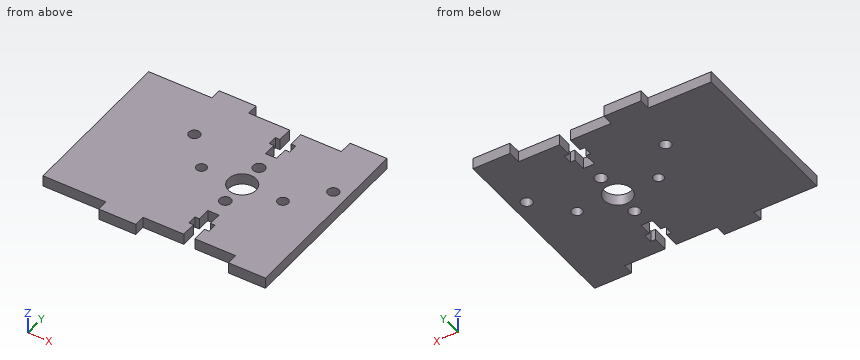
```python
from build123d import *

# Parameters (mm, degrees)
MODEL_R             = 3.750000001
MODEL_R_2           = 1.500000002
MODEL_R_3           = 1.353150001
MODEL_R_4           = 1.598250001
MODEL_R_5           = 1.533250001
MODEL_R_6           = 1.426350001
BOSS_EXTRUDE1_DEPTH = 3


with BuildPart() as part:
    # Model → Boss-Extrude1 (new body)
    with BuildSketch(Plane.XY):
        Polygon((58.24, 47.9), (61.24, 47.9), (61.24, 51.4001), (62.49, 51.4001), (62.49, 53.9001), (61.24, 53.9001), (61.24, 57.9), (72.24, 57.9), (72.24, 61.449728443), (82.24, 61.449728443), (82.24, 57.9), (82.24, 13.9), (82.24, 10.9), (72.24, 10.9), (72.24, 13.9), (61.24, 13.9), (61.24, 17.9), (62.49, 17.9), (62.49, 20.4), (61.24, 20.4), (61.24, 23.9), (58.24, 23.9), (58.24, 20.4), (56.99, 20.4), (56.99, 17.9), (58.24, 17.9), (58.24, 13.9), (47.24, 13.9), (47.24, 10.9), (37.24, 10.9), (37.24, 13.9), (20.24, 13.9), (20.24, 57.9), (37.24, 57.9), (37.24, 60.9), (47.24, 60.9), (47.24, 57.9), (58.24, 57.9), (58.24, 53.9001), (56.99, 53.9001), (56.99, 51.4001), (58.24, 51.4001), align=None)
        with Locations((59.739999999, 35.899999999)):
            Circle(MODEL_R, mode=Mode.SUBTRACT)
        with Locations((40.989999998, 44.899999998)):
            Circle(MODEL_R_2, mode=Mode.SUBTRACT)
        with Locations((48.73995, 35.90005)):
            Circle(MODEL_R_3, mode=Mode.SUBTRACT)
        with Locations((59.73995, 42.90005)):
            Circle(MODEL_R_4, mode=Mode.SUBTRACT)
        with Locations((59.73995, 28.90005)):
            Circle(MODEL_R_5, mode=Mode.SUBTRACT)
        with Locations((70.73995, 35.90005)):
            Circle(MODEL_R_6, mode=Mode.SUBTRACT)
        with Locations((78.489999998, 44.899999998)):
            Circle(MODEL_R_2, mode=Mode.SUBTRACT)
    extrude(amount=BOSS_EXTRUDE1_DEPTH)


solid = part.part
```
The model under review builds one solid part; all positions refer to its coordinate system, in mm. Round coordinates to 2 decimals unless told otherwise and drop trailing zeros. Loops run counter-clockwise (first coordinate to the right, second up) from the corner with the lowest first, then second, coordinate; pieces in that order, holes last. Notation, with made-up numbers: M 10,82 L 30,82 A19 ccw 30,90 Z; hole C 67.25,-5.75 d4. An arc over 180 degrees is marked long. Put each result on its own line as item: value.
Q1. To check wall thickness, follow L1, parallel to X at y = 35.9, z = 1.35; L2, parallel to X at y = 44.9, z = 0.85; L3, parallel to X at y = 22, z = 2.3. State the ranges of each line that lie inside material, in increasing order.
Result set:
L1: x = 20.24 to 47.39, 50.09 to 55.99, 63.49 to 69.31, 72.17 to 82.24
L2: x = 20.24 to 39.49, 42.49 to 76.99, 79.99 to 82.24
L3: x = 20.24 to 58.24, 61.24 to 82.24
Q2. Consider section B-B, the plane x = 59.74. Give the boundary of the cut face in (y, z), then the cut area to 3 significant figures.
Result set:
outline: M 23.9,0 L 27.37,0 L 27.37,3 L 23.9,3 Z; M 30.43,0 L 32.15,0 L 32.15,3 L 30.43,3 Z; M 39.65,0 L 41.3,0 L 41.3,3 L 39.65,3 Z; M 44.5,0 L 47.9,0 L 47.9,3 L 44.5,3 Z
area: 30.7 mm²
Q3. Consider section A-A, the plane x = 78.49. Give the boundary of the cut face in (y, z), then the cut area to 3 significant figures.
Result set:
outline: M 10.9,0 L 43.4,0 L 43.4,3 L 10.9,3 Z; M 46.4,0 L 61.45,0 L 61.45,3 L 46.4,3 Z
area: 143 mm²
Q4. Consider section D-D, the plane x = 53. Give the boundary of the cut face in (y, z).
Result set:
outline: M 13.9,0 L 57.9,0 L 57.9,3 L 13.9,3 Z
Q5. Consider section C-C, the plane y = 42. Give the boundary of the cut face in (x, z).
Result set:
outline: M 20.24,0 L 58.42,0 L 58.42,3 L 20.24,3 Z; M 61.06,0 L 82.24,0 L 82.24,3 L 61.06,3 Z
Q6. For pin 1 (1.5 mm diameter, centred on x = 69, z = 1.5, fed in from +Y); pin 2 (1.5 mm diameter, centred on x = 67, z = 1, fed in from -Y), all flat-tipped, find the tip position at first contact; note any pin that passes through.
Result set:
pin 1: stops at y = 57.9
pin 2: stops at y = 13.9
